Here's how the part is built. I have some questions about the finished solid (model axes, mm). A direction names the side the tool comes from. Round coordinates to 2 decimals unless told otherwise and drop trailing zeros. Order: outer loops, then holes, each group sorted by start corner. A loop starts at its lowest first (then second) coordinate and runs counter-clockwise, first axis right, second up. Notation, with made-up numbers: M -14.75,56.25 L 35.25,56.25 A36 cw 35.25,95.25 Z; hole C 49,62 d10. An arc over 180 degrees is marked long. Use one line per item in the form item = value. Start each with the question number.
```python
from build123d import *

# Parameters (mm, degrees)
SKETCH1_W           = 65.3
SKETCH1_H           = 46.5
BOSS_EXTRUDE1_DEPTH = 2.57
SKETCH2_R           = 1.6
CUT_EXTRUDE2_DEPTH  = 2.57
SKETCH3_R           = 5
CUT_EXTRUDE3_DEPTH  = 2.57
SKETCH4_W           = 5
SKETCH4_H           = 20
CUT_EXTRUDE4_DEPTH  = 10
FILLET1_R           = 2


with BuildPart() as part:
    # Sketch1 → Boss-Extrude1 (new body)
    with BuildSketch(Plane.XY):
        with Locations((-7.15, -18.05)):
            Rectangle(SKETCH1_W, SKETCH1_H)
    extrude(amount=BOSS_EXTRUDE1_DEPTH)

    # Sketch2 → Cut-Extrude2 (cut)
    with BuildSketch(Plane.XY.offset(2.57)):
        with Locations((15.7, -38.8)):
            Circle(SKETCH2_R)
        with Locations((15.7, 2.7)):
            Circle(SKETCH2_R)
        with Locations((-30, 2.7)):
            Circle(SKETCH2_R)
        with Locations((-30, -38.8)):
            Circle(SKETCH2_R)
    extrude(amount=-CUT_EXTRUDE2_DEPTH, mode=Mode.SUBTRACT)

    # Sketch3 → Cut-Extrude3 (cut)
    with BuildSketch(Plane.XY.offset(2.57)):
        with Locations((-39.8, -18.05)):
            Circle(SKETCH3_R)
    extrude(amount=-CUT_EXTRUDE3_DEPTH, mode=Mode.SUBTRACT)

    # Sketch4 → Cut-Extrude4 (cut)
    with BuildSketch(Plane.XY.offset(2.57)):
        with Locations((-37.3, -18.05)):
            Rectangle(SKETCH4_W, SKETCH4_H)
    extrude(amount=-CUT_EXTRUDE4_DEPTH, mode=Mode.SUBTRACT)

    # Fillet1
    fillet1_edges = [part.edges().sort_by_distance(p)[0] for p in [
        (-39.8, -8.05, 1.285),
        (-34.8, -28.05, 1.285),
        (-39.8, -28.05, 1.285),
        (-34.8, -8.05, 1.285),
    ]]
    fillet(fillet1_edges, radius=FILLET1_R)


solid = part.part
```
1) If we section it at C-C on z = 0.85: Write out the boundary of the cut face in (x, y), then the cut area to 3 significant figures.
2) If we section it at A-A on x = 15.7: Write out the boundary of the cut face in (y, z).
3) If we section it at B-B on y = -38.8: Write out the boundary of the cut face in (x, z).
4) If we section it at D-D on y = -17.5: Write out the boundary of the cut face in (x, z), then the cut area to 3 significant figures.
5) If I drill on line 1 (Y direction, x = 15.7, z = 1.8); line 2 (X direction, y = -11.5, z = 0.3), over which ranges is the centre line in solid material (lowest first)?
6) If we mould it in two halves opening along X, with no side actions, what happens to faces 3 (the flat face through (25.5, -18, 1)), 4 (the cylindrical face through (-39.23, -7.45, 1.27)), 5 (the cylindrical face through (17.226, 3.181, 1.303))? For each: +X half, -X half, draft (parallel to the pull), parting line (faces both ways), or undercut.
7) On a 3-axis mill with a long thin cutter (end or side, diameter ignored), from which of +Z, -Z, +X, -X, +Y, -Y can I reach the whole of each face in a straight line? I mean faces 1 (the flat face through (-39.8, -36, 1)), 2 (the flat face through (-34.8, -18, 1)). Say none if no direction works.
8) Will this pin go through, and if not, where does the flat tip stop? pin 1 Ø1.3 at (y, z) = (-21, 1) entering from -X.
Completed:
q1.outline = M -39.8,-41.3 L 25.5,-41.3 L 25.5,5.2 L -39.8,5.2 L -39.8,-6.05 A2 ccw -37.8,-8.05 L -36.8,-8.05 A2 cw -34.8,-10.05 L -34.8,-26.05 A2 cw -36.8,-28.05 L -37.8,-28.05 A2 ccw -39.8,-30.05 Z; hole C -30,-38.8 d3.2; hole C -30,2.7 d3.2; hole C 15.7,-38.8 d3.2; hole C 15.7,2.7 d3.2
q1.area = 2,900 mm²
q2.outline = M -41.3,0 L -40.4,0 L -40.4,2.57 L -41.3,2.57 Z; M -37.2,0 L 1.1,0 L 1.1,2.57 L -37.2,2.57 Z; M 4.3,0 L 5.2,0 L 5.2,2.57 L 4.3,2.57 Z
q3.outline = M -39.8,0 L -31.6,0 L -31.6,2.57 L -39.8,2.57 Z; M -28.4,0 L 14.1,0 L 14.1,2.57 L -28.4,2.57 Z; M 17.3,0 L 25.5,0 L 25.5,2.57 L 17.3,2.57 Z
q4.outline = M -34.8,0 L 25.5,0 L 25.5,2.57 L -34.8,2.57 Z
q4.area = 155 mm²
q5.line_1 = -41.3 to -40.4, -37.2 to 1.1, 4.3 to 5.2
q5.line_2 = -34.8 to 25.5
q6.face_3 = +X half
q6.face_4 = -X half
q6.face_5 = undercut
q7.face_1 = +Z, -Z, -X, +Y, -Y
q7.face_2 = +Z, -Z, -X
q8.pin_1 = -34.8
